Design review of the part shown in the three views and the two pictorial views. Dimensions are in mm from the part's minimum x, y and z. A direction names the side the tool comes from. Round coordinates to 2 decimals unless told otherwise and drop trailing zeros. Loops run counter-clockwise (first coordinate to the right, second up) from the corner with the lowest first, then second, coordinate; pieces in that order, holes last. Notation, with made-up numbers: (65.25, 29.25) -> (73.25, 29.25) arc R15 cw to (73.25, 47.25) -> close; hole circle Ø4 at (85.5, 65.5). An arc over 180 degrees is marked (long way). One line per question, with ' | ' between items. Start each with the question number.
1. For pin 1 Ø1.4 at (x, y) = (11, 1) entering from +Z; pin 2 Ø1.5 at (x, y) = (7, 0.5) entering from -Z; pin 3 Ø4 at (x, z) = (6, 6) entering from +Y, all flat-tipped, find the tip position at first contact; note any pin that passes through.
2. Consider section A-A (z = 8). Write out the cut boundary in (x, y).
3. Wall thickness on line 1 along Z through (x, y) = (17.5, 1.55); line 2 along Y through (x, z) = (3, 1.75); line 3 along X through (y, z) = (0.6, 6): over which ranges is each line inside the solid? List them lowest first.
4. Consider section B-B (x = 4.75). Write out the cut boundary in (y, z), and give its area (3 significant figures).
5. Consider section C-C (y = 0.75). Write out the cut boundary in (x, z).
6. Consider section D-D (x = 7). Write out the cut boundary in (y, z).
7. For the marked faces 1 and 2, list the 3-axis set-ups (+Z, -Z, +X, -X, +Y, -Y) from which the entire face can be reached by the end or side of a thin tool; tool diameter is ignored.
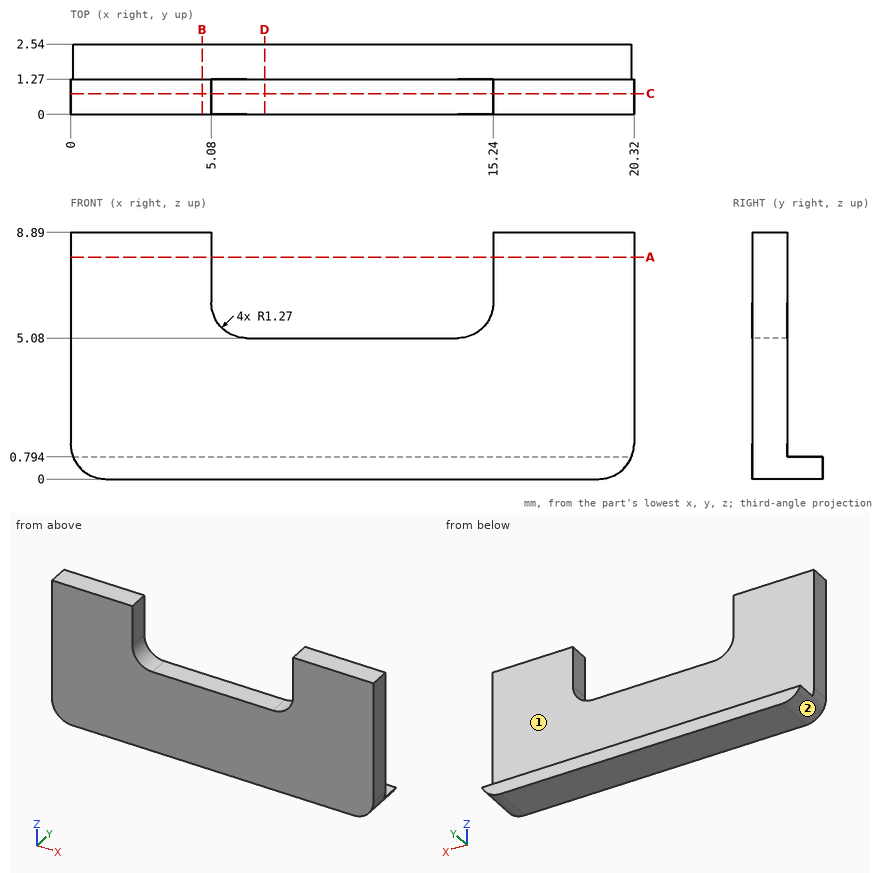
Answer block:
1) pin 1: stops at z = 5.08 | pin 2: stops at z = 0 | pin 3: stops at y = 1.27
2) outline: (0, 0) -> (5.08, 0) -> (5.08, 1.27) -> (0, 1.27) -> close; (15.24, 0) -> (20.32, 0) -> (20.32, 1.27) -> (15.24, 1.27) -> close
3) line 1: z = 0 to 0.79 | line 2: y = 0 to 1.27 | line 3: x = 0 to 5.13, 15.19 to 20.32
4) outline: (0, 0) -> (2.54, 0) -> (2.54, 0.79) -> (1.27, 0.79) -> (1.27, 8.89) -> (0, 8.89) -> close | area: 12.3 mm2
5) outline: (0, 1.27) arc R1.27 ccw to (1.27, 0) -> (19.05, 0) arc R1.27 ccw to (20.32, 1.27) -> (20.32, 8.89) -> (15.24, 8.89) -> (15.24, 6.35) arc R1.27 cw to (13.97, 5.08) -> (6.35, 5.08) arc R1.27 cw to (5.08, 6.35) -> (5.08, 8.89) -> (0, 8.89) -> close
6) outline: (0, 0) -> (2.54, 0) -> (2.54, 0.79) -> (1.27, 0.79) -> (1.27, 5.08) -> (0, 5.08) -> close
7) face 1: +Z, +X, -X, +Y | face 2: -Z, -X, +Y, -Y
